from build123d import *

# Parameters (mm, degrees)
F0_W     = 600
F0_H     = 575
F1_DEPTH = 18
F2_W     = 18
F2_H     = 50
F2_W_2   = 50
F2_H_2   = 18
F3_DEPTH = 10
F5_D     = 4.3
F6_D     = 4.3


with BuildPart() as f1:
    # F0 (on Top) → F1 (new body)
    with BuildSketch(Plane.XY):
        with Locations((300, -287.5)):
            Rectangle(F0_W, F0_H)
    extrude(amount=F1_DEPTH)

    # F2 (on face) → F3 (cut)
    with BuildSketch(Plane.XY.offset(18)):
        with Locations((39, -60)):
            Rectangle(F2_W, F2_H)
        with Locations((561, -60)):
            Rectangle(F2_W, F2_H)
        with Locations((561, -190)):
            Rectangle(F2_W, F2_H)
        with Locations((575, -259)):
            Rectangle(F2_W_2, F2_H_2)
        with Locations((25, -259)):
            Rectangle(F2_W_2, F2_H_2)
        with Locations((39, -190)):
            Rectangle(F2_W, F2_H)
    extrude(amount=-F3_DEPTH, mode=Mode.SUBTRACT)

    # F5 (through all)
    with Locations(Plane.XY.offset(18)):
        with Locations((200, -75), (222, -75), (200, -320), (222, -320), (378, -75), (400, -75), (400, -320), (378, -320), (378, -565), (400, -565), (200, -565), (222, -565)):
            Hole(F5_D / 2)

    # F6 (through all)
    with Locations(Plane.XY.offset(18)):
        with Locations((286, -76.75982), (314, -76.75982)):
            Hole(F6_D / 2)


solid = f1.part
Model file for the job. Use its own axes, mm. A direction names the side the tool comes from. Give positions to 0.01 mm unless a question says otherwise; leave off trailing zeros. Order: outer loops, then holes, each group sorted by start corner. A loop starts at its lowest first (then second) coordinate and runs counter-clockwise, first axis right, second up. Notation, with made-up numbers: (-34.75, 87) - (4.25, 87) arc R28 cw to (4.25, 108) - close; hole circle Ø3 at (24.25, 59). An arc over 180 degrees is marked (long way). Return JSON: item names as keys, results as strings.
1) Flat gauge pins, fed straight in: P1, Ø7, axis at x = 400, y = -565, coming from the -Z side; P2, Ø3.5, axis at x = 222, y = -320, coming from the +Z side; P3, Ø5.5, axis at x = 37.5, y = -54.5, coming from the +Z side. Where does each tip first touch, or does it go through?
Geometry says:
{"P1": "z = 0", "P2": "through", "P3": "z = 8"}
2) Cut at A-A, the plane y = -180. Give the cut face in (x, z).
Geometry says:
{"outline": "(0, 0) - (600, 0) - (600, 18) - (570, 18) - (570, 8) - (552, 8) - (552, 18) - (48, 18) - (48, 8) - (30, 8) - (30, 18) - (0, 18) - close"}
3) Probe line 1 (X direction, y = -204.5, z = 8.5); line 2 (Y direction, x = 222, z = 8.75); line 3 (X direction, y = -565, z = 10.25). List the from-to ranges inside material, lowest first. Write a range as from..to.
Geometry says:
{"line 1": "0..30, 48..552, 570..600", "line 2": "-575..-567.15, -562.85..-322.15, -317.85..-77.15, -72.85..0", "line 3": "0..197.85, 202.15..219.85, 224.15..375.85, 380.15..397.85, 402.15..600"}
4) 3-axis set-ups, long thin cutter, end or side, ignore diameter. For faces 1 (the flat face through (575, -259, 8)), 2 (the flat face through (561, -60, 8)), 3 (the flat face through (25, -259, 8)): which of +Z, -Z, +X, -X, +Y, -Y reach the whole face in a straight line?
Geometry says:
{"face 1": "+Z, +X", "face 2": "+Z", "face 3": "+Z, -X"}
5) Pull direction X, two halves, no side cores. Call faces 4 (the flat face through (296, -575, 9)), 5 (the flat face through (561, -190, 8)), 6 (the flat face through (600, -292, 9)): pulls with the +X half, pulls with the -X half, needs draft (parallel to the pull), parting line crosses it, or undercut.
Geometry says:
{"face 4": "needs draft", "face 5": "undercut", "face 6": "pulls with the +X half"}
